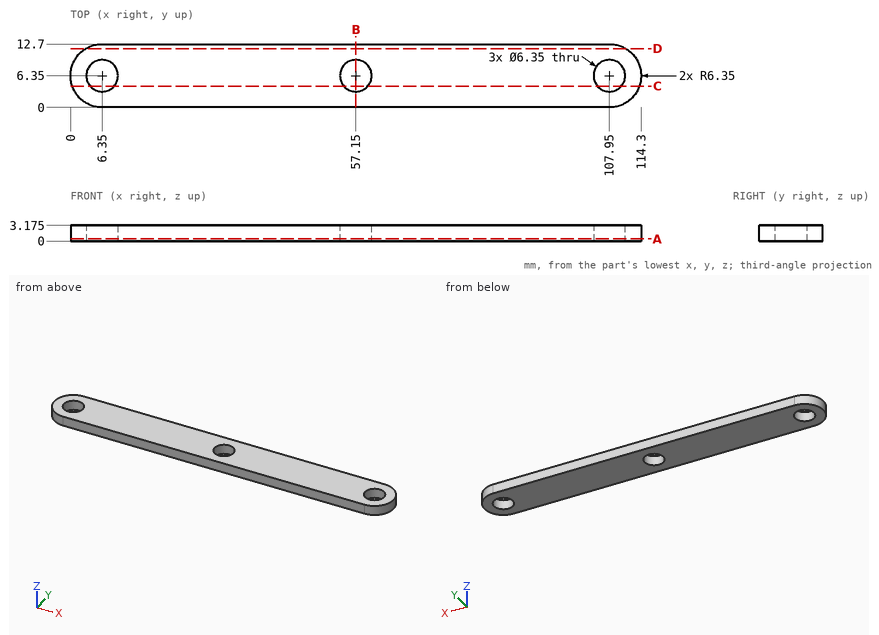
Geometry: see drawing. Coordinates: mm, zero at the bounding-box minimum. Coordinates: 2 decimals unless noted, no trailing zeros. Loops run counter-clockwise (first coordinate to the right, second up) from the corner with the lowest first, then second, coordinate; pieces in that order, holes last.
Q1. Cut plane D-D (y = 11.75). Output: boundary loops of the cut face in (x, z) (3 decimals).
Q2. Material intervals for line 1 (Y direction, x = 107.95, z = 1.05) (3 decimals); line 2 (X direction, y = 9.25, z = 2.3); line 3 (X direction, y = 6.75, z = 1.4), sorted ascending.
Q3. Cut plane B-B (x = 57.15). Output: boundary loops of the cut face in (y, z) (3 decimals), then the cut area to 3 significant figures.
Q4. Cut plane A-A (z = 0.5). Output: boundary loops of the cut face in (x, y) (3 decimals), then the cut area to 3 significant figures.
Q5. Contact query for a flat-ended pin moving along its axis: pin 1 (1 mm diameter, centred on y = 11.5, z = 2, fed in from +X). Output: stop coordinate, or through.
Q6. Cut plane C-C (y = 4.25). Output: boundary loops of the cut face in (x, z) (3 decimals).
Working result:
1. outline: (3.009, 0) - (111.291, 0) - (111.291, 3.175) - (3.009, 3.175) - close
2. line 1: y = 0 to 3.175, 9.525 to 12.7
2. line 2: x = 0.7 to 5.06, 7.64 to 55.86, 58.44 to 106.66, 109.24 to 113.6
2. line 3: x = 0.01 to 3.2, 9.5 to 54, 60.3 to 104.8, 111.1 to 114.29
3. outline: (0, 0) - (3.175, 0) - (3.175, 3.175) - (0, 3.175) - close; (9.525, 0) - (12.7, 0) - (12.7, 3.175) - (9.525, 3.175) - close
3. area: 20.2 mm2
4. outline: (6.35, 0) - (107.95, 0) arc R6.35 ccw to (107.95, 12.7) - (6.35, 12.7) arc R6.35 ccw to start; hole circle Ø6.35 at (6.35, 6.35); hole circle Ø6.35 at (57.15, 6.35); hole circle Ø6.35 at (107.95, 6.35)
4. area: 1,320 mm2
5. pin 1: stops at x = 112.27
6. outline: (0.357, 0) - (3.969, 0) - (3.969, 3.175) - (0.357, 3.175) - close; (8.731, 0) - (54.769, 0) - (54.769, 3.175) - (8.731, 3.175) - close; (59.531, 0) - (105.569, 0) - (105.569, 3.175) - (59.531, 3.175) - close; (110.331, 0) - (113.943, 0) - (113.943, 3.175) - (110.331, 3.175) - close
